Part model, mm, in its own coordinate system. A direction names the side the tool comes from. Give positions to 0.01 mm unless a question says otherwise; leave off trailing zeros. Write each loop counter-clockwise with the first axis right and the second up, starting at its lowest first coordinate (ties: lowest second). Pieces come first, ordered by that corner, then holes. Notation, with made-up numbers: M 14.5,60.25 L 67.5,60.25 A37 ccw 67.5,99.25 Z; hole C -34.5,-20 d3. An arc over 180 degrees is marked long. Use a Markdown table: item, result.
```python
from build123d import *

# Parameters (mm, degrees)
F0_R     = 11.5
F1_DEPTH = 38
F3_DEPTH = 23
F5_DEPTH = 19


with BuildPart() as f1:
    # F0 (on Top) → F1 (new body)
    with BuildSketch(Plane.XY):
        Circle(F0_R)
    extrude(amount=F1_DEPTH)

    # F2 (on face) → F3 (join)
    with BuildSketch(Plane.XY.offset(38)):
        Polygon((5.085656, 2.733027), (0.175957, 5.770821), (-4.909699, 3.037793), (-5.085656, -2.733027), (-0.175957, -5.770821), (4.909699, -3.037793), align=None)
    extrude(amount=F3_DEPTH)

    # F4 (on face) → F5 (cut)
    with BuildSketch(Plane(origin=(0, 0, 0), x_dir=(1, 0, 0), z_dir=(0, 0, -1))):
        Polygon((7.807994, -4.851312), (4.851312, 7.807994), (-7.807994, 4.851312), (-4.851312, -7.807994), align=None)
    extrude(amount=-F5_DEPTH, mode=Mode.SUBTRACT)


solid = f1.part
```
1. Cut at A-A, the plane y = 4.25. Give the cut face in (x, z), then the cut area to 3 significant figures.
Findings below:
| item | result |
|---|---|
| outline | M -10.69,0 L -5.68,0 L -5.68,19 L 7.67,19 L 7.67,0 L 10.69,0 L 10.69,38 L 2.63,38 L 2.63,61 L -2.65,61 L -2.65,38 L -10.69,38 Z |
| area | 680 mm2 |
2. Drill centre lines: L1, parallel to Z at x = 1.75, y = 2.25; L2, parallel to Z at x = -8.75, y = 4.25; L3, parallel to Y at x = 3.5, z = 5.5. Where is each one in solid material? Low to high.
Findings below:
| item | result |
|---|---|
| L1 | 19 to 61 |
| L2 | 0 to 38 |
| L3 | -10.95 to -7.49, 5.86 to 10.95 |
3. Cut at C-C, the plane z = 46.5. Give the cut face in (x, y).
Findings below:
| item | result |
|---|---|
| outline | M -5.09,-2.73 L -0.18,-5.77 L 4.91,-3.04 L 5.09,2.73 L 0.18,5.77 L -4.91,3.04 Z |
4. Two-plate mould, pull along Y, no slides. Class faces 1 (the flat face through (1.39, 6.35, 9.37)), 2 (the cylindrical face through (-1.5, 11.4, 18.7)), 3 (the flat face through (-2.67, -4.23, 49.34)): released by +Y, released by -Y, zero draft, split by the parting line, or undercut.
Findings below:
| item | result |
|---|---|
| face 1 | undercut |
| face 2 | split by the parting line |
| face 3 | released by -Y |
5. Cut at D-D, the plane x = -6. Give the cut face in (y, z).
Findings below:
| item | result |
|---|---|
| outline | M -9.81,0 L -5.27,0 L -5.27,19 L 2.89,19 L 2.89,0 L 9.81,0 L 9.81,38 L -9.81,38 Z |
6. Drop flat-ended pins along their axis: P1, Ø2, axis at x = -4.5, y = -6.5, coming from the +Z side; P2, Ø6, axis at x = 1.5, z = 15, coming from the -Y side; P3, Ø4.5, axis at x = -2, y = 1.5, coming from the -Z side; P4, Ø5, axis at y = 4, z = 7.5, coming from the -X side. Give the stop position or say it passes through.
Findings below:
| item | result |
|---|---|
| P1 | z = 38 |
| P2 | y = -11.5 |
| P3 | z = 19 |
| P4 | x = -11.4 |
7. Cut at B-B, the plane x = 4. Give the cut face in (y, z).
Findings below:
| item | result |
|---|---|
| outline | M -10.78,0 L -7.61,0 L -7.61,19 L 5.74,19 L 5.74,0 L 10.78,0 L 10.78,38 L 3.4,38 L 3.4,61 L -3.53,61 L -3.53,38 L -10.78,38 Z |
8. Tool access for faces 4 (the flat face through (2.331, -4.423, 49.339)), 5 (the flat face through (2, -5, 38)), 6 (the flat face through (2.67, 4.23, 49.34)), 7 (the flat face through (-2.331, 4.423, 49.339)), 8 (the flat face through (-6.35, 1.39, 9.37)): list every direction of +Z, -Z, +X, -X, +Y, -Y with a clear straight run to the whole face (end or side of a thin tool).
Findings below:
| item | result |
|---|---|
| face 4 | +Z, +X, -Y |
| face 5 | +Z |
| face 6 | +Z, +X, +Y |
| face 7 | +Z, -X, +Y |
| face 8 | -Z |
